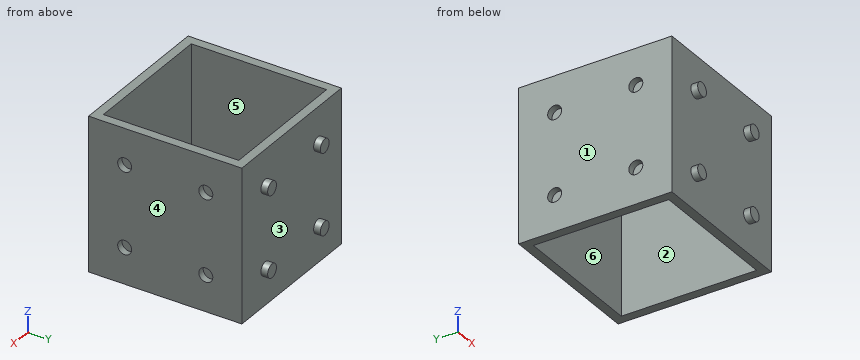
```python
from build123d import *

# Parameters (mm, degrees)
F0_W      = 170
F0_H      = 170
F1_DEPTH  = 85
F2_W      = 150
F2_H      = 150
F3_DEPTH  = 85
F7_R      = 7.5
F8_DEPTH  = 7.5
F6_R      = 7.5
F9_DEPTH  = 7.5
F5_R      = 7.75
F10_DEPTH = 7.5
F4_R      = 7.75
F11_DEPTH = 7.5


with BuildPart() as f1:
    # F0 (on Top) → F1 (new body, symmetric)
    with BuildSketch(Plane.XY):
        Rectangle(F0_W, F0_H)
    extrude(amount=F1_DEPTH, both=True)

    # F2 (on Top) → F3 (cut, symmetric)
    with BuildSketch(Plane.XY):
        Rectangle(F2_W, F2_H)
    extrude(amount=F3_DEPTH, both=True, mode=Mode.SUBTRACT)

    # F7 (on face) → F8 (join, symmetric)
    with BuildSketch(Plane.XZ.offset(85)):
        with Locations((-45, 45)):
            Circle(F7_R)
        with Locations((45, 45)):
            Circle(F7_R)
        with Locations((45, -45)):
            Circle(F7_R)
        with Locations((-45, -45)):
            Circle(F7_R)
    extrude(amount=F8_DEPTH, both=True)

    # F6 (on face) → F9 (join, symmetric)
    with BuildSketch(Plane(origin=(0, 85, 0), x_dir=(-1, 0, 0), z_dir=(0, 1, 0))):
        with Locations((45, -45)):
            Circle(F6_R)
        with Locations((45, 45)):
            Circle(F6_R)
        with Locations((-45, 45)):
            Circle(F6_R)
        with Locations((-45, -45)):
            Circle(F6_R)
    extrude(amount=F9_DEPTH, both=True)

    # F5 (on face) → F10 (cut, symmetric)
    with BuildSketch(Plane(origin=(-85, 0, 0), x_dir=(0, -1, 0), z_dir=(-1, 0, 0))):
        with Locations((-45, 45)):
            Circle(F5_R)
        with Locations((45, 45)):
            Circle(F5_R)
        with Locations((45, -45)):
            Circle(F5_R)
        with Locations((-45, -45)):
            Circle(F5_R)
    extrude(amount=F10_DEPTH, both=True, mode=Mode.SUBTRACT)

    # F4 (on face) → F11 (cut, symmetric)
    with BuildSketch(Plane.YZ.offset(85)):
        with Locations((-45, 45)):
            Circle(F4_R)
        with Locations((45, 45)):
            Circle(F4_R)
        with Locations((45, -45)):
            Circle(F4_R)
        with Locations((-45, -45)):
            Circle(F4_R)
    extrude(amount=F11_DEPTH, both=True, mode=Mode.SUBTRACT)


solid = f1.part
```
Can you work these out from the model? Positions are in its coordinate system, mm. Face numbers are marked on the shaded views. A direction names the side the tool comes from. Give positions to 0.01 mm unless a question says otherwise; leave off trailing zeros. Write each loop counter-clockwise with the first axis right and the second up, starting at its lowest first coordinate (ties: lowest second). Pieces come first, ordered by that corner, then holes. Notation, with made-up numbers: (20.25, -19.5) - (53.25, -19.5) arc R9 ccw to (53.25, -11.5) - close; hole circle Ø2 at (40.5, 41). An arc over 180 degrees is marked (long way). Write item = value, one per line. Start each with the question number.
1. On a 3-axis mill with a long thin cutter (end or side, diameter ignored), from which of +Z, -Z, +X, -X, +Y, -Y can I reach the whole of each face in a straight line? I mean the marked faces 1 and 2. Say none if no direction works.
2. Imagine slicing it at B-B (x = -2). Please give me the cut outline in (y, z).
3. For pin 1 (5 mm diameter, centred on x = 62, z = 30, fed in from -Y); pin 2 (9.5 mm diameter, centred on y = -45, z = 45, fed in from +X); pin 3 (2 mm diameter, centred on x = -4, z = -63.5, fed in from +Y), each with a flat end and sliding along its axis, tell me the tip position at first contact or that it passes through.
4. Imagine slicing it at C-C (z = 27). Please give me the cut outline in (x, y), and give its area (3 significant figures).
5. Please list where these lines run through material, in increasing order: line 1 (Z direction, x = 79, y = -45); line 2 (X direction, y = -30, z = -67).
6. Thinking about a two-plate mould opening in Y: for the marked faces 3, 4, 5 and 6, which applies, released by +Y, released by -Y, zero draft, split by the parting line, or undercut?
7. Imagine slicing it at A-A (y = -45). Please give me the cut outline in (x, z).
Worked answers:
q1.face_1 = +Z, -Z, -X, +Y, -Y
q1.face_2 = +Z, -Z
q2.outline = (-85, -85) - (-75, -85) - (-75, 85) - (-85, 85) - close; (75, -85) - (85, -85) - (85, 85) - (75, 85) - close
q3.pin_1 = -85
q3.pin_2 = 77.5
q3.pin_3 = 85
q4.outline = (-85, -85) - (85, -85) - (85, 85) - (-85, 85) - close; hole (-75, -75) - (75, -75) - (75, 75) - (-75, 75) - close
q4.area = 6,400 mm2
q5.line_1 = -85 to -52.75, -37.25 to 37.25, 52.75 to 85
q5.line_2 = -85 to -75, 75 to 85
q6.face_3 = released by +Y
q6.face_4 = zero draft
q6.face_5 = undercut
q6.face_6 = undercut
q7.outline = (-85, -85) - (-75, -85) - (-75, 85) - (-85, 85) - (-85, 52.75) - (-77.5, 52.75) - (-77.5, 37.25) - (-85, 37.25) - (-85, -37.25) - (-77.5, -37.25) - (-77.5, -52.75) - (-85, -52.75) - close; (75, -85) - (85, -85) - (85, -52.75) - (77.5, -52.75) - (77.5, -37.25) - (85, -37.25) - (85, 37.25) - (77.5, 37.25) - (77.5, 52.75) - (85, 52.75) - (85, 85) - (75, 85) - close
